Autodesk Inventor part; units mm, degrees
ref_plane "YZ Plane" through (0, 0, 0) normal (1, 0, 0) x (0, 1, 0)
ref_plane "XZ Plane" through (0, 0, 0) normal (0, 1, 0) x (-1, 0, 0)
ref_plane "XY Plane" through (0, 0, 0) normal (0, 0, 1) x (1, 0, 0)
sketch "Sketch1" plane through (0, 0, 0) normal (0, 0, 1) x (1, 0, 0)
  line L0 (0, 0) -> (6.35, 0)
  line L1 (0, 0) -> (-6.3448, 0)
  line L2 (6.35, 0) -> (82.5616, 131.9842)
  line L3 (82.5616, 131.9842) -> (69.8518, 131.9842)
  line L4 (69.8518, 131.9842) -> (0.0026, 10.9947)
  line L5 (0.0026, 10.9947) -> (-69.8461, 131.9845)
  line L6 (-6.3448, 0) -> (-82.5554, 131.9845)
  line L7 (-82.5554, 131.9845) -> (-69.8461, 131.9845)
  dimension "d2" = 6.35
extrude "Extrusion1" add sketch "Sketch1" along normal blind 12.7
sketch "Sketch2" plane through (-6.3448, 0, 0) normal (0, -1, 0) x (1, 0, 0)
  circle A0 centre (6.3474, 6.35) radius 38.1
  point P0 (6.3448, 0)
  dimension "d7" = 76.2
extrude "Extrusion2" add sketch "Sketch2" along normal blind 12.7
fillet "Fillet1" radius 12.7 1 edges at (-38.0974, 0, 6.35)
fillet "Fillet2" radius 2.8575 1 edges at (0.0026, 10.9947, 6.35)
sketch "Sketch4" plane through (0, 0, 12.7) normal (0, 0, 1) x (1, 0, 0)
  line L0 (82.5616, 131.9842) -> (69.8518, 131.9842) construction
  line L1 (69.8518, 131.9842) -> (2.4773, 15.2813) construction
  line L2 (63.5021, 120.9855) -> (63.5021, 131.9842)
  line L3 (63.5021, 131.9842) -> (57.7871, 131.9842)
  line L4 (57.7871, 131.9842) -> (57.7871, 111.0863)
  line L5 (-63.5021, 120.9855) -> (-63.5021, 131.9842)
  line L6 (-63.5021, 131.9842) -> (-57.7871, 131.9842)
  line L7 (-57.7871, 131.9842) -> (-57.7871, 111.0862)
  line L8 (-63.5021, 120.9855) -> (-57.7871, 111.0862)
  line L9 (-2.4721, 15.2813) -> (-69.8461, 131.9845)
  line L10 (57.7871, 111.0863) -> (63.5021, 120.9855)
  point P0 (0, 0)
  dimension "d19" = 12.7
  dimension "d20" = 5.715
extrude "Extrusion4" add sketch "Sketch4" against normal blind 12.7
fillet "Fillet5" radius 5.3975 2 edges at (57.7871, 131.9842, 6.35) (-57.7871, 131.9842, 6.35)
fillet "Fillet6" radius 13.335 2 edges at (69.8518, 131.9842, 6.35) (-69.8461, 131.9845, 6.35)
properties part number "mask holder" material "Rubber"
The model under review builds one solid part; all positions refer to its coordinate system, in mm. A direction names the side the tool comes from. Give positions to 0.01 mm unless a question says otherwise; leave off trailing zeros. Write each loop counter-clockwise with the first axis right and the second up, starting at its lowest first coordinate (ties: lowest second). Pieces come first, ordered by that corner, then holes. Notation, with made-up numbers: M 32,-13 L 46,-13 A28 ccw 46,15 Z; hole C 83.5,38.25 d2. An arc over 180 degrees is marked long. Write item = value, one per line. Start each with the question number.
Q1. We need section B-B (y = 74.5). State the section outline as (x, z) points, plus the area to 3 significant figures.
Q2. We need section C-C (y = 30). State the section outline as (x, z) points.
Q3. Mouldability with a two-part tool opening along X and no side actions: class faces 1 (the face through (-0.039, 13.853, 6.439)), 2 (the face through (-80, 131.984, 6)), 3 (the face through (-43.917, 65.068, 6.261)), 4 (the face through (59.326, 130.361, 6.261)) as released by +X, released by -X, zero draft, split by the parting line, or undercut.
Q4. Clearance check with flat-ended pins moving along their axes: pin 1 (6 mm diameter, centred on x = 16.5, z = 13.5, fed in from +Y); pin 2 (5.5 mm diameter, centred on y = 129, z = 8, fed in from +X); pin 3 (6 mm diameter, centred on x = 44, z = 3, fed in from +Y). State where each tip first meets the part, or that it passes through.
Q5. For line 1 (X direction, y = 123, z = 3); line 2 (Z direction, x = 36.5, y = 68); line 3 (Y direction, x = 17.5, z = 19.5), list the stretches that pass through material, from the lowest coordinate up.
Q6. Machinability: for faces 5 (the face through (80, 131.984, 6)), 6 (the face through (57.787, 119, 6)), 7 (the face through (43.922, 65.068, 6.261)), 8 (the face through (0, 0, -5)), which of the approach directions +Z, -Z, +X, -X, +Y, -Y give a long, thin tool a straight path to every point of the face, cutting with its end or side? Answer none if there is none.
Q7. We need section D-D (x = 55). State the section outline as (y, z) points.
Result set:
q1.outline = M -49.36,0 L -36.66,0 L -36.66,12.7 L -49.36,12.7 Z; M 36.67,0 L 49.37,0 L 49.37,12.7 L 36.67,12.7 Z
q1.area = 323 mm2
q2.outline = M -23.67,0 L -10.97,0 L -10.97,12.7 L -23.67,12.7 Z; M 10.97,0 L 23.67,0 L 23.67,12.7 L 10.97,12.7 Z
q3.face_1 = undercut
q3.face_2 = zero draft
q3.face_3 = released by -X
q3.face_4 = undercut
q4.pin_1 = 44.58
q4.pin_2 = 82.43
q4.pin_3 = 92.4
q5.line_1 = -77.37 to -64.66, -63.5 to -57.79, 57.79 to 63.5, 64.67 to 77.37
q5.line_2 = 0 to 12.7
q5.line_3 = -12.7 to 0
q6.face_5 = +Z, -Z, +X, -X, +Y
q6.face_6 = +Z, -Z, +Y
q6.face_7 = +Z, -Z, +X
q6.face_8 = none
q7.outline = M 84.25,0 L 106.26,0 L 106.26,12.7 L 84.25,12.7 Z
